Could you check a few things on this model? Use its own coordinates, in mm. Face numbers are marked on the shaded views. Coordinates: 2 decimals unless noted, no trailing zeros. Loops run counter-clockwise (first coordinate to the right, second up) from the corner with the lowest first, then second, coordinate; pieces in that order, holes last. Notation, with made-up numbers: (9, 6.25) - (46, 6.25) arc R22 ccw to (46, 13.25) - close; hole circle Ø7 at (46.25, 63). An arc over 180 degrees is marked (long way). One line per item, written item: value. Start each with the question number.
(1) If I drill on line 1 along Y through (x, z) = (19.5, -33); line 2 along Y through (x, z) = (28, 17); line 3 along Z through (x, y) = (25.5, -2.5), over which ranges is the centre line in solid material (lowest first)? Write a range as from..to.
(2) I'm going to push flat-ended pins straight in: P1, Ø0.9, axis at x = 14, z = -33, coming from the +Y side; P2, Ø3, axis at x = 31.5, y = -4.5, coming from the -Z side; P3, Ø6, axis at x = 13.5, z = -0.5, coming from the +Y side. Where does each tip first touch, or does it pass through?
(3) If we section it at B-B on y = -20: Write out the boundary of the cut face in (x, z), then the cut area to 3 significant figures.
(4) If we section it at D-D on y = 6: Write out the boundary of the cut face in (x, z).
(5) If we section it at A-A on x = 6.5: Write out the boundary of the cut face in (y, z), then the cut area to 3 significant figures.
(6) If we section it at C-C on z = -16: Write out the boundary of the cut face in (x, y).
(7) If we mould it in two halves opening along Z, with no side actions, what happens to the marked faces 1, 2 and 3? For each: pulls with the +Z half, pulls with the -Z half, needs draft (parallel to the pull), parting line crosses it, or undercut.
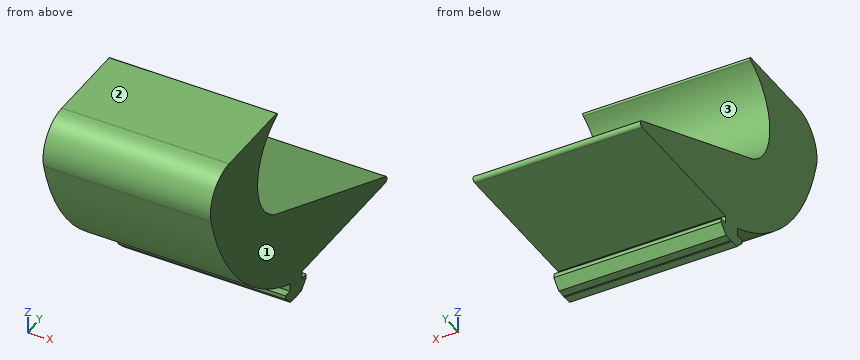
```python
from build123d import *

# Parameters (mm, degrees)
BOSS_EXTRUDE1_DEPTH = 50
FILLET1_R           = 1
FILLET2_R           = 0.5
BOSS_EXTRUDE2_DEPTH = 50
FILLET3_R           = 70
FILLET4_R           = 10


with BuildPart() as part:
    # Sketch1 → Boss-Extrude1 (new body)
    with BuildSketch(Plane(origin=(0, 0, 0), x_dir=(0, 0, -1), z_dir=(1, 0, 0))):
        with BuildLine():
            Line((-30, -50), (30, -50))
            Line((30, -50), (30, 50))
            Line((30, 50), (2.079852522, -13.995823026))
            ThreePointArc((2.079852522, -13.995823026), (-15.294169853, -22.708497617), (-30, -10))
            Line((-30, -10), (-30, -50))
        make_face()
    extrude(amount=BOSS_EXTRUDE1_DEPTH)

    # Fillet1
    fillet1_edges = [part.edges().sort_by_distance(p)[0] for p in [
        (25, 50, -30),
    ]]
    fillet(fillet1_edges, radius=FILLET1_R)

    # Fillet2
    fillet2_edges = [part.edges().sort_by_distance(p)[0] for p in [
        (25, -10, 30),
    ]]
    fillet(fillet2_edges, radius=FILLET2_R)

    # Sketch2 → Boss-Extrude2 (add)
    with BuildSketch(Plane(origin=(50, 0, 0), x_dir=(0, 0, -1), z_dir=(1, 0, 0))):
        Polygon((31.455, 0.728575996), (30, 0.728575996), (30, -5.521424004), (31.455, -5.521424004), (31.8, -5.521424004), (32.3, -5.521424004), (32.3, -7.896424004), (33.439339828, -7.896424004), (36.1, -5.235763833), (36.1, -2.606424004), (36.31, -2.396424004), (36.1, -2.186424004), (36.1, 0.442915824), (33.439339828, 3.103575996), (32.3, 3.103575996), (32.3, 0.728575996), (31.8, 0.728575996), align=None)
    extrude(amount=-BOSS_EXTRUDE2_DEPTH)

    # Fillet3
    # the kernel refuses this fillet: 70 mm, written as the material it takes off along each edge
    with BuildSketch(Plane(origin=(-162.95430565, -50, -30), x_dir=(0, 0, 1), z_dir=(1, 0, 0))) as fillet3_piece_1:
        with BuildLine():
            CenterArc((65.18172226, -70), FILLET3_R, 90, 68.617538212)
            Line((0, -44.478575996), (0, 0))
            Line((0, 0), (65.18172226, 0))
        make_face()
    extrude(amount=375.9086113, mode=Mode.SUBTRACT)

    # Fillet4
    fillet4_edges = [part.edges().sort_by_distance(p)[0] for p in [
        (25, -49.807949078, 30),
    ]]
    fillet(fillet4_edges, radius=FILLET4_R)


solid = part.part
```
Values:
1. line 1: y = -7.9..3.1
1. line 2: y = -47.6..-22.41
1. line 3: z = -36.21..-7.1
2. P1: stops at y = 3.1
2. P2: stops at z = -36.1
2. P3: stops at y = -10.74
3. outline: (0, -22.26) - (50, -22.26) - (50, 3.57) - (0, 3.57) - close; (0, 22.69) - (50, 22.69) - (50, 30) - (0, 30) - close
3. area: 1,660 mm2
4. outline: (0, -30) - (50, -30) - (50, -10.8) - (0, -10.8) - close
5. outline: (-47.72, 17.47) arc R70 ccw to (-5.52, -30) - (-5.52, -32.3) - (-7.9, -32.3) - (-7.9, -33.44) - (-5.24, -36.1) - (-2.61, -36.1) - (-2.4, -36.31) - (-2.19, -36.1) - (0.44, -36.1) - (3.1, -33.44) - (3.1, -32.3) - (0.73, -32.3) - (0.73, -30) - (45.21, -30) arc R1 ccw to (45.61, -28.08) - (-14, -2.08) arc R17.5 cw to (-12.62, 29.05) arc R0.5 ccw to (-12.83, 30) - (-38.05, 30) arc R10 ccw to start
5. area: 2,080 mm2
6. outline: (0, -27.75) - (50, -27.75) - (50, 17.91) - (0, 17.91) - close
7. face 1: needs draft
7. face 2: pulls with the +Z half
7. face 3: undercut
